Could you check a few things on this drawing? It's one solid part, dimensions in mm from its lowest x, y, z. A direction names the side the tool comes from. Give positions to 0.01 mm unless a question says otherwise; leave off trailing zeros. Loops run counter-clockwise (first coordinate to the right, second up) from the corner with the lowest first, then second, coordinate; pieces in that order, holes last. Notation, with made-up numbers: (47.5, 9.5) - (58.5, 9.5) arc R21 ccw to (58.5, 34.5) - close; hole circle Ø4 at (67.5, -28.5). An arc over 180 degrees is marked (long way). Use a Markdown table: item, result.
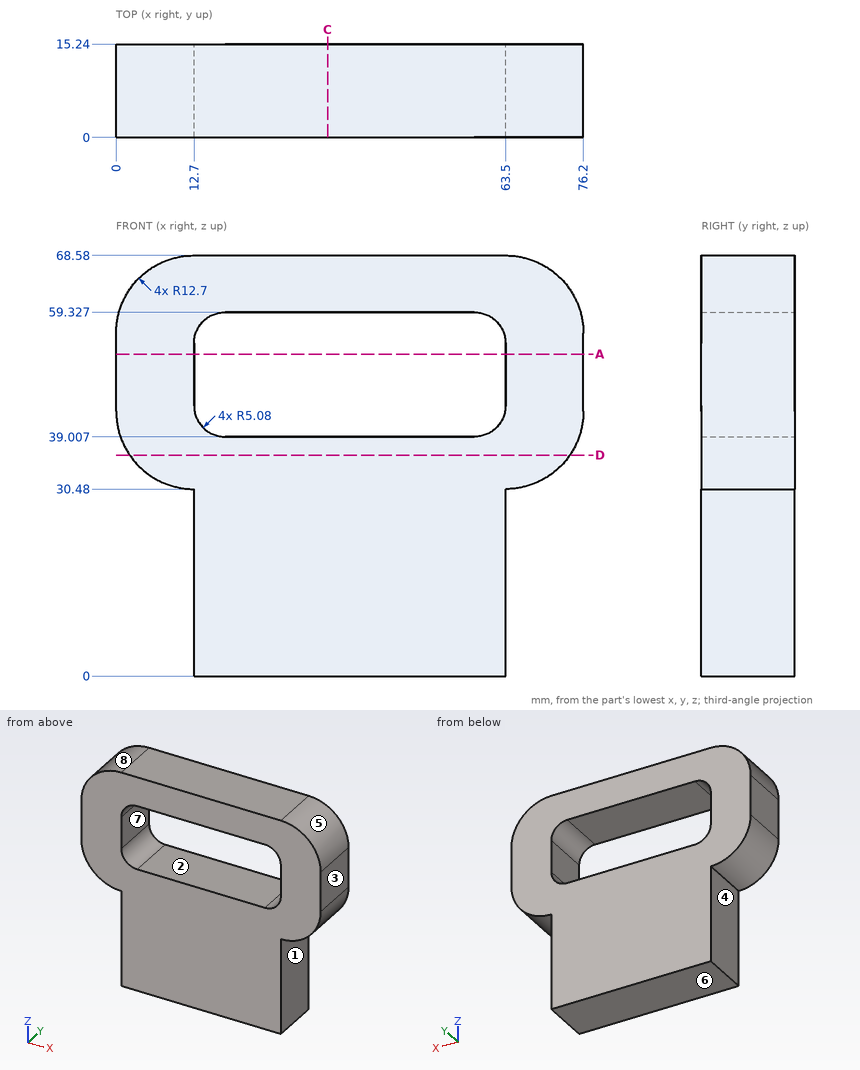
(1) On a 3-axis mill with a long thin cutter (end or side, diameter ignored), from which of +Z, -Z, +X, -X, +Y, -Y can I reach the whole of each face in a straight line? I mean the marked faces 1, 2, 3 and 4. Say none if no direction works.
A:
| item | result |
|---|---|
| face 1 | -Z, +X, +Y, -Y |
| face 2 | +Y, -Y |
| face 3 | +Z, -Z, +X, +Y, -Y |
| face 4 | -Z, -X, +Y, -Y |
(2) Suppose I cut it at C-C on x = 34.5. Write out the boundary of the cut face in (y, z).
A:
| item | result |
|---|---|
| outline | (0, 0) - (15.24, 0) - (15.24, 39.01) - (0, 39.01) - close; (0, 59.33) - (15.24, 59.33) - (15.24, 68.58) - (0, 68.58) - close |
(3) Suppose I cut it at A-A on z = 52.5. Write out the boundary of the cut face in (x, y).
A:
| item | result |
|---|---|
| outline | (0, 0) - (12.7, 0) - (12.7, 15.24) - (0, 15.24) - close; (63.5, 0) - (76.2, 0) - (76.2, 15.24) - (63.5, 15.24) - close |
(4) We'd pull the mould along X, two halves only. Please class the marked faces 5, 6, 7 and 8: pulls with the +X half, pulls with the -X half, needs draft (parallel to the pull), parting line crosses it, or undercut.
A:
| item | result |
|---|---|
| face 5 | pulls with the +X half |
| face 6 | needs draft |
| face 7 | undercut |
| face 8 | pulls with the -X half |
(5) Will this pin go through, and if not, where does the flat tip stop? pin 1 (4 mm diameter, centred on y = 3.5, z = 16.5, fed in from +X).
A:
| item | result |
|---|---|
| pin 1 | x = 63.5 |
(6) Suppose I cut it at D-D on z = 36. Write out the boundary of the cut face in (x, y).
A:
| item | result |
|---|---|
| outline | (2.22, 0) - (73.98, 0) - (73.98, 15.24) - (2.22, 15.24) - close |
(7) If I drill on line 1 (X direction, y = 6.5, z = 50.5); line 2 (Z direction, x = 27, y = 9.25); line 3 (X direction, y = 0.75, z = 57.5) (1 decimal), over which ranges is the centre line in solid material (lowest first)?
A:
| item | result |
|---|---|
| line 1 | 0 to 12.7, 63.5 to 76.2 |
| line 2 | 0 to 39.01, 59.33 to 68.58 |
| line 3 | 0.1 to 13.9, 62.3 to 76.1 |
